```python
from build123d import *

# Parameters (mm, degrees)
SKETCH1_W           = 25
SKETCH1_H           = 24
SKETCH1_R           = 1
BOSS_EXTRUDE1_DEPTH = 1
SKETCH2_W           = 8
SKETCH2_H           = 8
BOSS_EXTRUDE2_DEPTH = 4
SKETCH3_R           = 4
BOSS_EXTRUDE3_DEPTH = 1
FILLET2_R           = 0.5
SKETCH4_W           = 16
SKETCH4_H           = 5
BOSS_EXTRUDE4_DEPTH = 2
FILLET3_R           = 0.5
SKETCH5_R           = 3.5
CUT_EXTRUDE1_DEPTH  = 6
BOSS_EXTRUDE5_DEPTH = 1
SKETCH7_W           = 0.2
SKETCH7_H           = 4.34
CUT_EXTRUDE2_DEPTH  = 1
LPATTERN1_COUNT     = 14
LPATTERN1_PITCH     = 0.3


with BuildPart() as part:
    # Sketch1 → Boss-Extrude1 (new body)
    with BuildSketch(Plane.XY):
        Rectangle(SKETCH1_W, SKETCH1_H)
        with Locations((10.5, 10)):
            Circle(SKETCH1_R, mode=Mode.SUBTRACT)
        with Locations((-10.5, 10)):
            Circle(SKETCH1_R, mode=Mode.SUBTRACT)
        with Locations((-10.5, -2.5)):
            Circle(SKETCH1_R, mode=Mode.SUBTRACT)
        with Locations((10.5, -2.5)):
            Circle(SKETCH1_R, mode=Mode.SUBTRACT)
    extrude(amount=BOSS_EXTRUDE1_DEPTH)

    # Sketch2 → Boss-Extrude2 (add)
    with BuildSketch(Plane.XY.offset(1)):
        with Locations((0, -2.5)):
            Rectangle(SKETCH2_W, SKETCH2_H)
    extrude(amount=BOSS_EXTRUDE2_DEPTH)

    # Sketch3 → Boss-Extrude3 (add)
    with BuildSketch(Plane.XY.offset(5)):
        with Locations((0, -2.5)):
            Circle(SKETCH3_R)
    extrude(amount=BOSS_EXTRUDE3_DEPTH)

    # Fillet2
    fillet2_edges = [part.edges().sort_by_distance(p)[0] for p in [
        (4, -2.5, 1),
        (-4, -2.5, 1),
        (0, -6.5, 1),
    ]]
    fillet(fillet2_edges, radius=FILLET2_R)

    # Sketch4 → Boss-Extrude4 (add)
    with BuildSketch(Plane(origin=(0, 0, 0), x_dir=(-1, 0, 0), z_dir=(0, 0, -1))):
        with Locations((0, -7.5)):
            Rectangle(SKETCH4_W, SKETCH4_H)
    extrude(amount=BOSS_EXTRUDE4_DEPTH)

    # Fillet3
    fillet3_edges = [part.edges().sort_by_distance(p)[0] for p in [
        (-8, -7.5, 0),
        (-8, -10, -1),
        (0, -5, 0),
        (-8, -5, -1),
        (8, -7.5, 0),
        (8, -5, -1),
        (0, -10, 0),
        (8, -10, -1),
        (-8, -7.5, -2),
        (0, -5, -2),
        (8, -7.5, -2),
        (0, -10, -2),
    ]]
    fillet(fillet3_edges, radius=FILLET3_R)

    # Sketch5 → Cut-Extrude1 (cut)
    with BuildSketch(Plane.XY.offset(6)):
        with Locations((0, -2.5)):
            Circle(SKETCH5_R)
    extrude(amount=-CUT_EXTRUDE1_DEPTH, mode=Mode.SUBTRACT)

    # Sketch6 → Boss-Extrude5 (add)
    with BuildSketch(Plane.XY.offset(1)):
        Polygon((-3.152517362, 10.68), (-3.152517362, 5.84), (-2.322578899, 5.84), (-2.322578899, 1.5), (2.017421101, 1.5), (2.017421101, 5.84), (2.846354447, 5.84), (2.846354447, 6.468877905), (2.846354447, 10.68), align=None)
    extrude(amount=BOSS_EXTRUDE5_DEPTH)

    # Sketch7 → Cut-Extrude2 (cut)
    with BuildSketch(Plane.XY.offset(2)):
        with Locations((-2.072578899, 3.67)):
            Rectangle(SKETCH7_W, SKETCH7_H)
    cut_extrude2 = extrude(amount=-CUT_EXTRUDE2_DEPTH, mode=Mode.SUBTRACT)

    # LPattern1: Cut-Extrude2 ×14
    with Locations(*[(i * LPATTERN1_PITCH, 0, 0) for i in range(1, LPATTERN1_COUNT)]):
        add(cut_extrude2, mode=Mode.SUBTRACT)


solid = part.part
```
Could you check a few things on this model? Use its own coordinates, in mm. A direction names the side the tool comes from. Coordinates: 2 decimals unless noted, no trailing zeros. Write each loop counter-clockwise with the first axis right and the second up, starting at its lowest first coordinate (ties: lowest second). Pieces come first, ordered by that corner, then holes. Notation, with made-up numbers: (67.5, 81) -> (71.5, 81) arc R24 ccw to (71.5, 99) -> close; hole circle Ø2 at (62, 57.25). An arc over 180 degrees is marked (long way). Return JSON: item names as keys, results as strings.
(1) Which directions (+Z, -Z, +X, -X, +Y, -Y) give clear straight access to the entire face, cutting with the end or side of a thin tool? Please do faces 1 (the flat face through (-2.7, 5.84, 1.5)), 2 (the flat face through (-8, -8, -1)), 3 (the flat face through (4, -3, 3)), 4 (the flat face through (8, -8, -1)).
Numbers:
{"face 1": "+Z, -X", "face 2": "-Z, -X, +Y, -Y", "face 3": "+Z, +X, +Y, -Y", "face 4": "-Z, +X, +Y, -Y"}
(2) Imagine slicing it at A-A, the plane y = 10. Please give me the cut outline in (x, z), then the cut area to 3 significant figures.
Numbers:
{"outline": "(-12.5, 0) -> (-11.5, 0) -> (-11.5, 1) -> (-12.5, 1) -> close; (-9.5, 0) -> (9.5, 0) -> (9.5, 1) -> (2.85, 1) -> (2.85, 2) -> (-3.15, 2) -> (-3.15, 1) -> (-9.5, 1) -> close; (11.5, 0) -> (12.5, 0) -> (12.5, 1) -> (11.5, 1) -> close", "area": "27.0 mm2"}
(3) I'm going to push flat-ended pins straight in: pin 1 (1 mm diameter, centred on x = 3, y = 1.5, fed in from +Z); pin 2 (0.8 mm diameter, centred on y = 4, z = 1.5, fed in from +X); pin 3 (3 mm diameter, centred on x = 10.5, y = -2.5, fed in from +Z); pin 4 (2 mm diameter, centred on y = 3, z = -0.5, fed in from +X). Where does each tip first touch, or does it pass through?
Numbers:
{"pin 1": "stops at z = 5", "pin 2": "stops at x = 2.02", "pin 3": "stops at z = 1", "pin 4": "stops at x = 12.5"}
(4) Imagine slicing it at D-D, the plane y = -3. Count the separate pieces of the cut face and the enclosed holes in it, then the cut area to 3 significant figures.
Numbers:
{"separate pieces": "4", "enclosed holes": "0", "area": "20.0 mm2"}
(5) Imagine slicing it at B-B, the plane x = 10.5. Please give me the cut outline in (y, z), then the cut area to 3 significant figures.
Numbers:
{"outline": "(-12, 0) -> (-3.5, 0) -> (-3.5, 1) -> (-12, 1) -> close; (-1.5, 0) -> (9, 0) -> (9, 1) -> (-1.5, 1) -> close; (11, 0) -> (12, 0) -> (12, 1) -> (11, 1) -> close", "area": "20.0 mm2"}
(6) I need wall thicknesses on L1, parallel to Y at x = -10.5, z = 0.35; L2, parallel to Y at x = 2.75, z = 1.5; L3, parallel to Z at x = 8.75, y = 5.25. Which ranges of each line are inside material? Lowest first, please.
Numbers:
{"L1": "y = -12 to -3.5, -1.5 to 9, 11 to 12", "L2": "y = -6.5 to -4.67, -0.33 to 1.5, 5.84 to 10.68", "L3": "z = 0 to 1"}
(7) Imagine slicing it at C-C, the plane z = 4. Please give me the cut outline in (x, y), then the cut area to 3 significant figures.
Numbers:
{"outline": "(-4, -6.5) -> (4, -6.5) -> (4, 1.5) -> (-4, 1.5) -> close; hole circle Ø7 at (0, -2.5)", "area": "25.5 mm2"}
(8) We'd pull the mould along Y, two halves only. Please class faces 5 (the cylindrical face through (10.37, 10.99, 0.49)), 6 (the flat face through (-0.2, -12, 0.5)), 7 (the flat face through (-3.153, 8.3, 1.5)): +Y half, -Y half, draft (parallel to the pull), parting line (faces both ways), or undercut.
Numbers:
{"face 5": "undercut", "face 6": "-Y half", "face 7": "draft"}
